Here's how the part is built. I have some questions about the finished solid (model axes, mm). Round coordinates to 2 decimals unless told otherwise and drop trailing zeros. Loops run counter-clockwise (first coordinate to the right, second up) from the corner with the lowest first, then second, coordinate; pieces in that order, holes last. Notation, with made-up numbers: M 44.5,-8 L 95.5,-8 A15 ccw 95.5,2 Z; hole C 78.5,-1 d4. An arc over 180 degrees is marked long. Use a Markdown table: item, result.
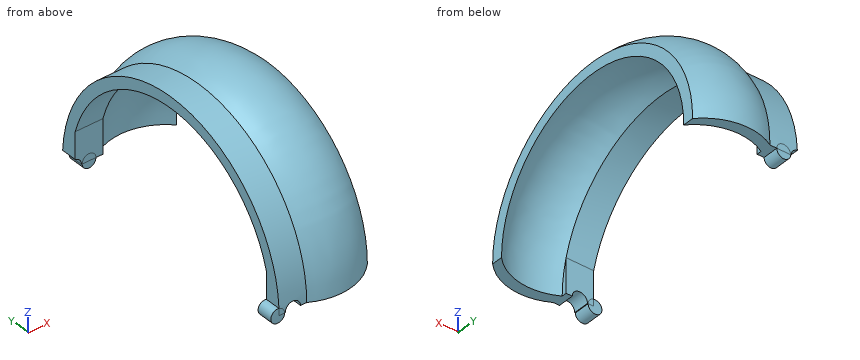
```python
from build123d import *

# Parameters (mm, degrees)
REVOLVE1_ANGLE           = 180
BOSS_EXTRUDE1_DEPTH      = 20
BOSS_EXTRUDE2_REACH      = 228.274
BOSS_EXTRUDE2_END_RADIUS = 97.5
SKETCH5_R                = 5
CUT_EXTRUDE1_REACH       = 228.274
CUT_EXTRUDE1_END_RADIUS  = 97.5
SKETCH6_R                = 5.5
BOSS_EXTRUDE3_REACH      = 228.274
BOSS_EXTRUDE3_END_RADIUS = 97.5
SKETCH8_R                = 5
CUT_EXTRUDE2_REACH       = 228.274
CUT_EXTRUDE2_END_RADIUS  = 97.5
SKETCH10_R               = 5.5


with BuildPart() as part:
    # Sketch1 → Revolve1 (revolve)
    with BuildSketch(Plane.XY):
        with BuildLine():
            Line((0, 89.5), (20, 89.5))
            ThreePointArc((20, 89.5), (46.3125, 94.5), (70, 82))
            Line((70, 82), (70, 90))
            ThreePointArc((70, 90), (46.3125, 102.5), (20, 97.5))
            Line((20, 97.5), (0, 97.5))
            Line((0, 97.5), (0, 89.5))
        make_face()
    revolve(axis=Axis((0, 0, 0), (1, 0, 0)), revolution_arc=REVOLVE1_ANGLE)

    # Sketch3 → Boss-Extrude1 (add)
    with BuildSketch(Plane.ZY):
        with BuildLine():
            ThreePointArc((24.784067463, 86), (12.514991011, 88.620680431), (0, 89.5))
            Line((0, 89.5), (0, 86))
            Line((0, 86), (24.784067463, 86))
        make_face()
        with BuildLine():
            Line((0, -86), (0, -89.5))
            ThreePointArc((0, -89.5), (12.514991011, -88.620680431), (24.784067463, -86))
            Line((24.784067463, -86), (0, -86))
        make_face()
    extrude(amount=-BOSS_EXTRUDE1_DEPTH)

    # Boss-Extrude2: up to this cylinder (the profile starts inside it)
    boss_extrude2_end = Plane(origin=(10, 0, 0), z_dir=(-1, 0, 0)) * Cylinder(BOSS_EXTRUDE2_END_RADIUS, 652.548, mode=Mode.PRIVATE)
    # Sketch5 → Boss-Extrude2 (add, up to the surface)
    with BuildSketch(Plane.XZ.offset(-86), mode=Mode.PRIVATE) as boss_extrude2_sk1:
        with Locations((10, 0)):
            Circle(SKETCH5_R)
    boss_extrude2_tool1 = extrude(boss_extrude2_sk1.sketch, amount=-BOSS_EXTRUDE2_REACH, mode=Mode.PRIVATE) & boss_extrude2_end
    add(boss_extrude2_tool1.solids().sort_by_distance((10, 86, 0))[0])

    # Cut-Extrude1: up to this cylinder (the profile starts inside it)
    cut_extrude1_end = Plane(origin=(10, 0, 0), z_dir=(-1, 0, 0)) * Cylinder(CUT_EXTRUDE1_END_RADIUS, 652.548, mode=Mode.PRIVATE)
    # Sketch6 → Cut-Extrude1 (cut, up to the surface)
    with BuildSketch(Plane(origin=(0, -86, 0), x_dir=(1, 0, 0), z_dir=(0, 1, 0)), mode=Mode.PRIVATE) as cut_extrude1_sk1:
        with Locations((10, 0)):
            Circle(SKETCH6_R)
    cut_extrude1_tool1 = extrude(cut_extrude1_sk1.sketch, amount=-CUT_EXTRUDE1_REACH, mode=Mode.PRIVATE) & cut_extrude1_end
    add(cut_extrude1_tool1.solids().sort_by_distance((10, -86, 0))[0], mode=Mode.SUBTRACT)

    # Boss-Extrude3: up to this cylinder (the profile starts inside it)
    boss_extrude3_end = Plane(origin=(-1, 0, 0), z_dir=(-1, 0, 0)) * Cylinder(BOSS_EXTRUDE3_END_RADIUS, 652.548, mode=Mode.PRIVATE)
    # Sketch8 → Boss-Extrude3 (add, up to the surface)
    with BuildSketch(Plane(origin=(0, -86, 0), x_dir=(1, 0, 0), z_dir=(0, 1, 0)), mode=Mode.PRIVATE) as boss_extrude3_sk1:
        with Locations((-1, 0)):
            Circle(SKETCH8_R)
    boss_extrude3_tool1 = extrude(boss_extrude3_sk1.sketch, amount=-BOSS_EXTRUDE3_REACH, mode=Mode.PRIVATE) & boss_extrude3_end
    add(boss_extrude3_tool1.solids().sort_by_distance((-1, -86, 0))[0])

    # Cut-Extrude2: up to this cylinder (the profile starts inside it)
    cut_extrude2_end = Plane(origin=(-1, 0, 0), z_dir=(-1, 0, 0)) * Cylinder(CUT_EXTRUDE2_END_RADIUS, 652.548, mode=Mode.PRIVATE)
    # Sketch10 → Cut-Extrude2 (cut, up to the surface)
    with BuildSketch(Plane.XZ.offset(-86), mode=Mode.PRIVATE) as cut_extrude2_sk1:
        with Locations((-1, 0)):
            Circle(SKETCH10_R)
    cut_extrude2_tool1 = extrude(cut_extrude2_sk1.sketch, amount=-CUT_EXTRUDE2_REACH, mode=Mode.PRIVATE) & cut_extrude2_end
    add(cut_extrude2_tool1.solids().sort_by_distance((-1, 86, 0))[0], mode=Mode.SUBTRACT)


solid = part.part
```
Q1. Will these pins go through, and if not, where does the flat tip stop? P1, Ø6, axis at x = 32.5, y = 54.5, coming from the +Z side; P2, Ø2, axis at x = 46.5, y = -70, coming from the +Z side; P3, Ø16, axis at x = 10.5, z = 7.5, coming from the +Y side.
Return value:
| item | result |
|---|---|
| P1 | stops at z = 88.38 |
| P2 | stops at z = 75.78 |
| P3 | stops at y = 97.5 |
Q2. I need wall thicknesses on line 1 (Y direction, x = 2, z = 27.5); line 2 (Y direction, x = 5.5, z = 21); line 3 (Z direction, x = 8.5, y = -43). Which ranges of each line are inside material? Lowest first, please. Write a range as from..to.
Return value:
| item | result |
|---|---|
| line 1 | y = -93.54..-85.17, 85.17..93.54 |
| line 2 | y = -95.21..-86, 86..95.21 |
| line 3 | z = 78.49..87.51 |
Q3. Imagine slicing it at B-B, the plane x = 30. Please give me the cut outline in (y, z), then the cut area to 3 significant figures.
Return value:
| item | result |
|---|---|
| outline | M -101.62,0 L -93.62,0 A93.62 cw 93.62,0 L 101.62,0 A101.62 ccw Z |
| area | 2,450 mm^2 |
